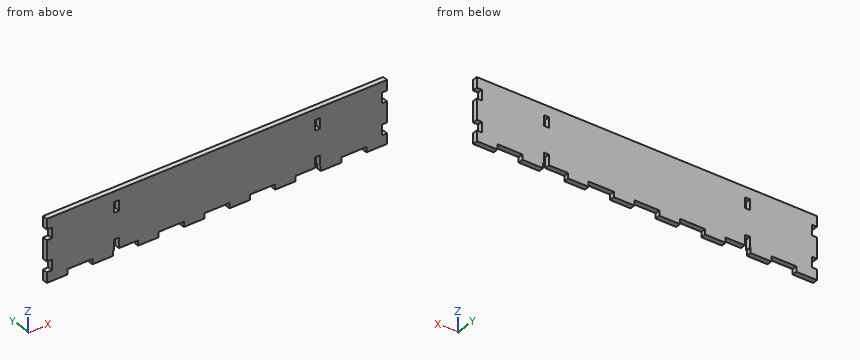
```python
from build123d import *

# Parameters (mm, degrees)
F0_W     = 419.1
F0_H     = 76.2
F1_DEPTH = 6.35
F2_W     = 30.842857
F2_H     = 6.35
F2_W_2   = 30.842858
F2_W_3   = 6.35
F2_H_2   = 12.7
F3_DEPTH = 6.351
F4_W     = 6.35
F4_H     = 12.7
F5_DEPTH = 6.351


with BuildPart() as f1:
    # F0 (on Front) → F1 (new body)
    with BuildSketch(Plane.XZ):
        Rectangle(F0_W, F0_H)
    extrude(amount=F1_DEPTH)

    # F2 (on face) → F3 (cut, through all)
    with BuildSketch(Plane.XZ.offset(6.35)):
        with Locations((-168.728571, -34.925)):
            Rectangle(F2_W, F2_H)
        with Locations((-112.485715, -34.925)):
            Rectangle(F2_W, F2_H)
        with Locations((-56.242857, -34.925)):
            Rectangle(F2_W, F2_H)
        with Locations((0, -34.925)):
            Rectangle(F2_W_2, F2_H)
        with Locations((56.242857, -34.925)):
            Rectangle(F2_W, F2_H)
        with Locations((112.485715, -34.925)):
            Rectangle(F2_W, F2_H)
        with Locations((168.728571, -34.925)):
            Rectangle(F2_W, F2_H)
        with Locations((-206.375, -19.05)):
            Rectangle(F2_W_3, F2_H_2)
        with Locations((-206.375, 19.05)):
            Rectangle(F2_W_3, F2_H_2)
        with Locations((206.375, 19.05)):
            Rectangle(F2_W_3, F2_H_2)
        with Locations((206.375, -19.05)):
            Rectangle(F2_W_3, F2_H_2)
    extrude(amount=-F3_DEPTH, mode=Mode.SUBTRACT)

    # F4 (on face) → F5 (cut, through all)
    with BuildSketch(Plane.XZ.offset(6.35)):
        with Locations((-123.825, -25.4)):
            Rectangle(F4_W, F4_H)
        with Locations((-123.825, 19.05)):
            Rectangle(F4_W, F4_H)
        with Locations((123.825, 19.05)):
            Rectangle(F4_W, F4_H)
        with Locations((123.825, -25.4)):
            Rectangle(F4_W, F4_H)
    extrude(amount=-F5_DEPTH, mode=Mode.SUBTRACT)


solid = f1.part
```
Model file for the job. Use its own axes, mm. Coordinates: 2 decimals unless noted, no trailing zeros. Order: outer loops, then holes, each group sorted by start corner. A loop starts at its lowest first (then second) coordinate and runs counter-clockwise, first axis right, second up. Notation, with made-up numbers: M 41,-19 L 53,-19 A27 cw 53,8 Z; hole C 57.5,-30 d11. An arc over 180 degrees is marked long. Answer as CSV lines item,"result".
(1) Wall check: line 1 along X through (y, z) = (-1, 14.5); line 2 along Z through (x, y) = (-159, -3.25); line 3 along X through (y, z) = (-2, -14). Give the ranges that are in metal, low to high.
Geometry says:
line 1,"x = -203.2 to -127, -120.65 to 120.65, 127 to 203.2"
line 2,"z = -31.75 to 38.1"
line 3,"x = -203.2 to 203.2"
(2) Band-saw the part on B-B, the plane x = -108.5. List the corners of the cut face in (y, z), then the cut area to 3 significant figures.
Geometry says:
outline,"M -6.35,-31.75 L 0,-31.75 L 0,38.1 L -6.35,38.1 Z"
area,"444 mm2"
(3) Band-saw the part on A-A, the plane y = -2. State how many separate pieces and enclosed holes the cut face has, then the cut area to 3 significant figures.
Geometry says:
separate pieces,"1"
enclosed holes,"2"
area,"29,900 mm2"
(4) Flat gauge pins, fed straight in: pin 1 (3 mm diameter, centred on y = -1, z = -19.5, fed in from +X); pin 2 (3 mm diameter, centred on x = 123.5, y = -3.5, fed in from -Z). Where does each tip first touch, or does it go through?
Geometry says:
pin 1,"stops at x = 203.2"
pin 2,"stops at z = -19.05"
